Geometry: final body of the model. Coordinates: model frame, mm. A direction names the side the tool comes from. Round coordinates to 2 decimals unless told otherwise and drop trailing zeros. Loops run counter-clockwise (first coordinate to the right, second up) from the corner with the lowest first, then second, coordinate; pieces in that order, holes last. Notation, with made-up numbers: M 83.25,-30.75 L 93.25,-30.75 A4 ccw 93.25,-25.75 Z; hole C 57,-15.5 d10. An arc over 180 degrees is marked long. Answer as a JSON object with one key per item and string values.
```python
from build123d import *

# Parameters (mm, degrees)
SKETCH1_W                    = 514.4008
SKETCH1_H                    = 103.2002
BOSS_EXTRUDE1_DEPTH          = 1.6002
CONVERT_SOLID1_OUTLINE_W     = 514.4008
CONVERT_SOLID1_OUTLINE_H     = 103.2002
CONVERT_SOLID1_DEPTH         = 0.6858
EDGE_FLANGE1_STRIP_W         = 5.4864
EDGE_FLANGE1_STRIP_H         = 0.9144
EDGE_FLANGE1_STRIP_CUT_DEPTH = 103.2002
EDGE_FLANGE1_DEPTH           = 103.2002
EDGE_FLANGE2_STRIP_W         = 5.4864
EDGE_FLANGE2_STRIP_H         = 0.9144
EDGE_FLANGE2_STRIP_CUT_DEPTH = 103.2002
EDGE_FLANGE2_DEPTH           = 103.2002
CUT_EXTRUDE3_DEPTH           = 521.084421643
CUT_EXTRUDE3_DEPTH_BACK      = 521.084421643
SKETCH18_R                   = 3.2639
EDGE_FLANGE3_STRIP_W         = 5.4864
EDGE_FLANGE3_STRIP_H         = 0.9144
EDGE_FLANGE3_STRIP_CUT_DEPTH = 512.572
EDGE_FLANGE3_DEPTH           = 512.572
SKETCH22_R                   = 3.2639
CUT_EXTRUDE4_DEPTH           = 2.54


# Read off the part's stored shape, not the designer's step: Convert-Solid1
# Sheet-metal steps are written as plain solids
with BuildPart() as part:
    # Sketch1 → Boss-Extrude1 (new body)
    with BuildSketch(Plane.XY):
        Rectangle(SKETCH1_W, SKETCH1_H)
    extrude(amount=BOSS_EXTRUDE1_DEPTH)

    # Convert-Solid1 outline → Convert-Solid1 (cut)
    with BuildSketch(Plane.XY):
        Rectangle(CONVERT_SOLID1_OUTLINE_W, CONVERT_SOLID1_OUTLINE_H)
    extrude(amount=CONVERT_SOLID1_DEPTH, mode=Mode.SUBTRACT)

    # Edge-Flange1 strip (across the edge) → Edge-Flange1 strip cut (cut)
    with BuildSketch(Plane(origin=(257.2004, 51.6001, 0.6858), x_dir=(-1, 0, 0), z_dir=(0, -1, 0))):
        with Locations((-1.8288, -0.4572)):
            Rectangle(EDGE_FLANGE1_STRIP_W, EDGE_FLANGE1_STRIP_H)
    extrude(amount=EDGE_FLANGE1_STRIP_CUT_DEPTH, mode=Mode.SUBTRACT)

    # Edge-Flange1 section (across the edge) → Edge-Flange1 (add)
    with BuildSketch(Plane(origin=(257.2004, 51.6001, 0.6858), x_dir=(-1, 0, 0), z_dir=(0, -1, 0))):
        with BuildLine():
            Line((-0.9144, 0.9144), (-0.9144, 37.1856))
            Line((-0.9144, 37.1856), (0, 37.1856))
            Line((0, 37.1856), (0, 0.9144))
            ThreePointArc((0, 0.9144), (0.267821559, 0.267821559), (0.9144, 0))
            Line((0.9144, 0), (0.9144, -0.9144))
            ThreePointArc((0.9144, -0.9144), (-0.378756881, -0.378756881), (-0.9144, 0.9144))
        make_face()
    extrude(amount=EDGE_FLANGE1_DEPTH)

    # Edge-Flange2 strip (across the edge) → Edge-Flange2 strip cut (cut)
    with BuildSketch(Plane(origin=(-257.2004, -51.6001, 0.6858), x_dir=(1, 0, 0), z_dir=(0, 1, 0))):
        with Locations((-1.8288, -0.4572)):
            Rectangle(EDGE_FLANGE2_STRIP_W, EDGE_FLANGE2_STRIP_H)
    extrude(amount=EDGE_FLANGE2_STRIP_CUT_DEPTH, mode=Mode.SUBTRACT)

    # Edge-Flange2 section (across the edge) → Edge-Flange2 (add)
    with BuildSketch(Plane(origin=(-257.2004, -51.6001, 0.6858), x_dir=(1, 0, 0), z_dir=(0, 1, 0))):
        with BuildLine():
            Line((-0.9144, 0.9144), (-0.9144, 37.1856))
            Line((-0.9144, 37.1856), (0, 37.1856))
            Line((0, 37.1856), (0, 0.9144))
            ThreePointArc((0, 0.9144), (0.267821559, 0.267821559), (0.9144, 0))
            Line((0.9144, 0), (0.9144, -0.9144))
            ThreePointArc((0.9144, -0.9144), (-0.378756881, -0.378756881), (-0.9144, 0.9144))
        make_face()
    extrude(amount=EDGE_FLANGE2_DEPTH)

    # Sketch18 → Cut-Extrude3 (cut, two sides: drawn at the far end of the back side and taken through both)
    with BuildSketch(Plane.ZY.offset(258.1148).offset(-CUT_EXTRUDE3_DEPTH_BACK)):
        with Locations(Location((-19.244729261, 26.2001, 0), (0, 0, 180))):
            Circle(SKETCH18_R)
        with Locations(Location((-19.244729261, -26.2001, 0), (0, 0, 180))):
            Circle(SKETCH18_R)
    extrude(amount=CUT_EXTRUDE3_DEPTH + CUT_EXTRUDE3_DEPTH_BACK, mode=Mode.SUBTRACT)

    # Edge-Flange3 strip (across the edge) → Edge-Flange3 strip cut (cut)
    with BuildSketch(Plane(origin=(-256.286, 51.6001, 0.6858), x_dir=(0, -1, 0), z_dir=(1, 0, 0))):
        with Locations((-1.8288, -0.4572)):
            Rectangle(EDGE_FLANGE3_STRIP_W, EDGE_FLANGE3_STRIP_H)
    extrude(amount=EDGE_FLANGE3_STRIP_CUT_DEPTH, mode=Mode.SUBTRACT)

    # Edge-Flange3 section (across the edge) → Edge-Flange3 (add)
    with BuildSketch(Plane(origin=(-256.286, 51.6001, 0.6858), x_dir=(0, -1, 0), z_dir=(1, 0, 0))):
        with BuildLine():
            Line((-0.9144, 0.9144), (-0.9144, 37.1856))
            Line((-0.9144, 37.1856), (0, 37.1856))
            Line((0, 37.1856), (0, 0.9144))
            ThreePointArc((0, 0.9144), (0.267821559, 0.267821559), (0.9144, 0))
            Line((0.9144, 0), (0.9144, -0.9144))
            ThreePointArc((0.9144, -0.9144), (-0.378756881, -0.378756881), (-0.9144, 0.9144))
        make_face()
    extrude(amount=EDGE_FLANGE3_DEPTH)

    # Sketch22 → Cut-Extrude4 (cut)
    with BuildSketch(Plane(origin=(0, 52.5145, 0), x_dir=(1, 0, 0), z_dir=(0, 1, 0))):
        with Locations(Location((230.886, 19.2786, 0), (0, 0, 270))):
            Circle(SKETCH22_R)
        with Locations(Location((115.443, 19.2786, 0), (0, 0, 270))):
            Circle(SKETCH22_R)
        with Locations(Location((0, 19.2786, 0), (0, 0, 270))):
            Circle(SKETCH22_R)
        with Locations(Location((-115.443, 19.2786, 0), (0, 0, 270))):
            Circle(SKETCH22_R)
        with Locations(Location((-230.886, 19.2786, 0), (0, 0, 270))):
            Circle(SKETCH22_R)
    extrude(amount=-CUT_EXTRUDE4_DEPTH, mode=Mode.SUBTRACT)


solid = part.part
```
1) First-contact query: pin 1 (5 mm diameter, centred on y = 26.2, z = -19.24, fed in from -X); pin 2 (7.5 mm diameter, centred on x = -115.44, z = -19.28, fed in from -Y); pin 3 (10 mm diameter, centred on x = -10, y = 33.5, fed in from -Z). Flat tips, straight axial feed; report the tip coordinate or a pass-through.
Geometry results:
{"pin 1": "through", "pin 2": "y = 51.6", "pin 3": "z = 0.69"}
2) Cut plane C-C on y = -5.5. Return the cut outline in (x, z).
Geometry results:
{"outline": "M -258.11,-36.5 L -257.2,-36.5 L -257.2,-0.23 A0.91 cw -256.29,0.69 L 256.29,0.69 A0.91 cw 257.2,-0.23 L 257.2,-36.5 L 258.11,-36.5 L 258.11,-0.23 A1.83 ccw 256.29,1.6 L -256.29,1.6 A1.83 ccw -258.11,-0.23 Z"}
3) Cut plane B-B on x = 77. Return the cut outline in (y, z).
Geometry results:
{"outline": "M -51.6,0.69 L 50.69,0.69 A0.91 cw 51.6,-0.23 L 51.6,-36.5 L 52.51,-36.5 L 52.51,-0.23 A1.83 ccw 50.69,1.6 L -51.6,1.6 Z"}
4) Line query: probe 1 along X at (y, z) = (13, -8.5); probe 2 along Z at (x, y) = (135, 38); probe 3 along Y at (x, z) = (-99.5, -26.5). Output: solid intervals per line, ascending.
Geometry results:
{"probe 1": "-258.11 to -257.2, 257.2 to 258.11", "probe 2": "0.69 to 1.6", "probe 3": "51.6 to 52.51"}
5) Pull-direction query (X, two-part tool) for faces 4 (the face through (-258.115, -1, -18)), 5 (the face through (-4, 51.6, -19)), 6 (the face through (-4, 52.514, -18)); classes: +X half, -X half, draft (parallel to the pull), parting line (faces both ways), or undercut.
Geometry results:
{"face 4": "-X half", "face 5": "undercut", "face 6": "draft"}
6) Set-up query: faces 1 (the face through (-4, 0, 1.6)), 2 (the face through (-257.2, -1, -19)), 3 (the face through (-4, 0, 0.686)). Return all of +Z, -Z, +X, -X, +Y, -Y with unobstructed straight access to the full face (end or side cutting, diameter ignored); none if empty.
Geometry results:
{"face 1": "+Z, +X, -X, +Y, -Y", "face 2": "-Z, +Y, -Y", "face 3": "-Z, -Y"}
7) Cut plane A-A on z = -29.5. Return the cut outline in (x, y), and give its area (3 significant figures).
Geometry results:
{"outline": "M -258.11,-51.6 L -257.2,-51.6 L -257.2,51.6 L -258.11,51.6 Z; M -256.29,51.6 L 256.29,51.6 L 256.29,52.51 L -256.29,52.51 Z; M 257.2,-51.6 L 258.11,-51.6 L 258.11,51.6 L 257.2,51.6 Z", "area": "657 mm2"}
